from build123d import *

# Parameters (mm, degrees)
F1_DEPTH = 25.4
F3_D     = 4.4
F4_R     = 3.96875
F5_DEPTH = 25.4
F6_R     = 5.08
F7_R     = 1.524


with BuildPart() as f1:
    # F0 (on Right) → F1 (new body)
    with BuildSketch(Plane.YZ):
        Polygon((-50.8, 7), (-50.8, 0), (0, 0), (0, 76.2), (-12, 76.2), (-12, 7), align=None)
    extrude(amount=F1_DEPTH)

    # F3 (through all)
    with Locations(Plane.XY.offset(7)):
        with Locations((20.32, -17.08), (5.08, -17.08), (5.08, -45.72), (20.32, -45.72)):
            Hole(F3_D / 2)

    # F4 (on face) → F5 (cut)
    with BuildSketch(Plane.XZ.offset(12)):
        with Locations((12.7, 57.8)):
            Circle(F4_R)
    extrude(amount=-F5_DEPTH, mode=Mode.SUBTRACT)

    # F6
    f6_edges = [f1.edges().sort_by_distance(p)[0] for p in [
        (25.4, -6, 76.2),
        (0, -6, 76.2),
        (25.4, -50.8, 3.5),
        (0, -50.8, 3.5),
    ]]
    fillet(f6_edges, radius=F6_R)

    # F7
    f7_edges = [f1.edges().sort_by_distance(p)[0] for p in [
        (12.7, -12, 7),
        (8.73125, -12, 57.8),
        (8.73125, 0, 57.8),
    ]]
    fillet(f7_edges, radius=F7_R)


solid = f1.part
Input: part model. Units: mm. Frame: model coordinates. A direction names the side the tool comes from. Round coordinates to 2 decimals unless told otherwise and drop trailing zeros. Loops run counter-clockwise (first coordinate to the right, second up) from the corner with the lowest first, then second, coordinate; pieces in that order, holes last. Notation, with made-up numbers: (20, 35) -> (32, 35) arc R20 ccw to (32, 48) -> close; hole circle Ø6 at (39, 14.25). An arc over 180 degrees is marked (long way). Answer as a JSON object with one key per item and string values. Group by question number.
1) Ray query, L1, parallel to Y at x = 20.32, z = 1.75; L2, parallel to Y at x = 22.25, z = 59; L3, parallel to Z at x = 7.75, y = -15.5. Return the intervals inside material, ascending.
2) Section query B-B on z = 57.8. Output: boundary loops of the cut face in (x, y), plus the area to 3 significant figures.
3) Section query A-A on x = 12.7. Output: boundary loops of the cut face in (y, z), plus the area to 3 significant figures.
4) Section query D-D on x = 4.25. Output: boundary loops of the cut face in (y, z), plus the area to 3 significant figures.
5) Draft query along X for faces 1 (the flat face through (25.4, -9, 28)), 2 (the flat face through (13, -6, 76.2)), 3 (the cylindrical face through (5.557, -19.228, 3.451)). Return one class per face: +X half, -X half, draft (parallel to the pull), parting line (faces both ways), or undercut.
6) Reachability of faces 4 (the flat face through (13, -32, 7)), 5 (the flat face through (13, 0, 38)) from +Z, -Z, +X, -X, +Y, -Y: full face, straight path, thin tool, end or side. Return the list, or none.
7) Section query C-C on y = -17.08. Output: boundary loops of the cut face in (x, z).
8) Pin query (flat end, axial travel): pin 1 (12.5 mm diameter, centred on x = 12.7, z = 57.8, fed in from -Y); pin 2 (12 mm diameter, centred on x = 15.5, y = -39, fed in from +Z); pin 3 (10 mm diameter, centred on x = 5, y = -18, fed in from +Z). Return the tip coordinate at first contact, or that it passes through.
Reply:
{
 "1": {"L1": "y = -50.8 to -47.92, -43.52 to -19.28, -14.88 to 0", "L2": "y = -12 to 0", "L3": "z = 0 to 7"},
 "2": {"outline": "(0, -12) -> (7.21, -12) arc R1.52 ccw to (8.73, -10.48) -> (8.73, -1.52) arc R1.52 ccw to (7.21, 0) -> (0, 0) -> close; (16.67, -10.48) arc R1.52 ccw to (18.19, -12) -> (25.4, -12) -> (25.4, 0) -> (18.19, 0) arc R1.52 ccw to (16.67, -1.52) -> close", "area": "208 mm2"},
 "3": {"outline": "(-50.8, 0) -> (0, 0) -> (0, 52.31) arc R1.52 ccw to (-1.52, 53.83) -> (-10.48, 53.83) arc R1.52 ccw to (-12, 52.31) -> (-12, 8.52) arc R1.52 cw to (-13.52, 7) -> (-50.8, 7) -> close; (-12, 63.29) arc R1.52 ccw to (-10.48, 61.77) -> (-1.52, 61.77) arc R1.52 ccw to (0, 63.29) -> (0, 76.2) -> (-12, 76.2) -> close", "area": "1,090 mm2"},
 "4": {"outline": "(-50.73, 0) -> (-47.76, 0) -> (-47.76, 7) -> (-50.73, 7) -> close; (-43.68, 0) -> (-19.12, 0) -> (-19.12, 7) -> (-43.68, 7) -> close; (-15.04, 0) -> (0, 0) -> (0, 76.13) -> (-12, 76.13) -> (-12, 8.52) arc R1.52 cw to (-13.52, 7) -> (-15.04, 7) -> close", "area": "1,130 mm2"},
 "5": {"face 1": "+X half", "face 2": "draft", "face 3": "undercut"},
 "6": {"face 4": "+Z, +X, -X, -Y", "face 5": "+Z, -Z, +X, -X, +Y"},
 "7": {"outline": "(0, 0) -> (2.88, 0) -> (2.88, 7) -> (0, 7) -> close; (7.28, 0) -> (18.12, 0) -> (18.12, 7) -> (7.28, 7) -> close; (22.52, 0) -> (25.4, 0) -> (25.4, 7) -> (22.52, 7) -> close"},
 "8": {"pin 1": "stops at y = -12", "pin 2": "stops at z = 7", "pin 3": "stops at z = 7.09"}
}
